Can you work these out from the drawing? Everything is in mm from the part's minimum corner. A direction names the side the tool comes from. Round coordinates to 2 decimals unless told otherwise and drop trailing zeros. Order: outer loops, then holes, each group sorted by start corner. A loop starts at its lowest first (then second) coordinate and runs counter-clockwise, first axis right, second up. Notation, with made-up numbers: (88.5, 17) - (129.5, 17) arc R13 cw to (129.5, 40) - close; hole circle Ø4 at (36.5, 2.25). An arc over 180 degrees is marked (long way). Answer as a JSON object with one key per item and string values.
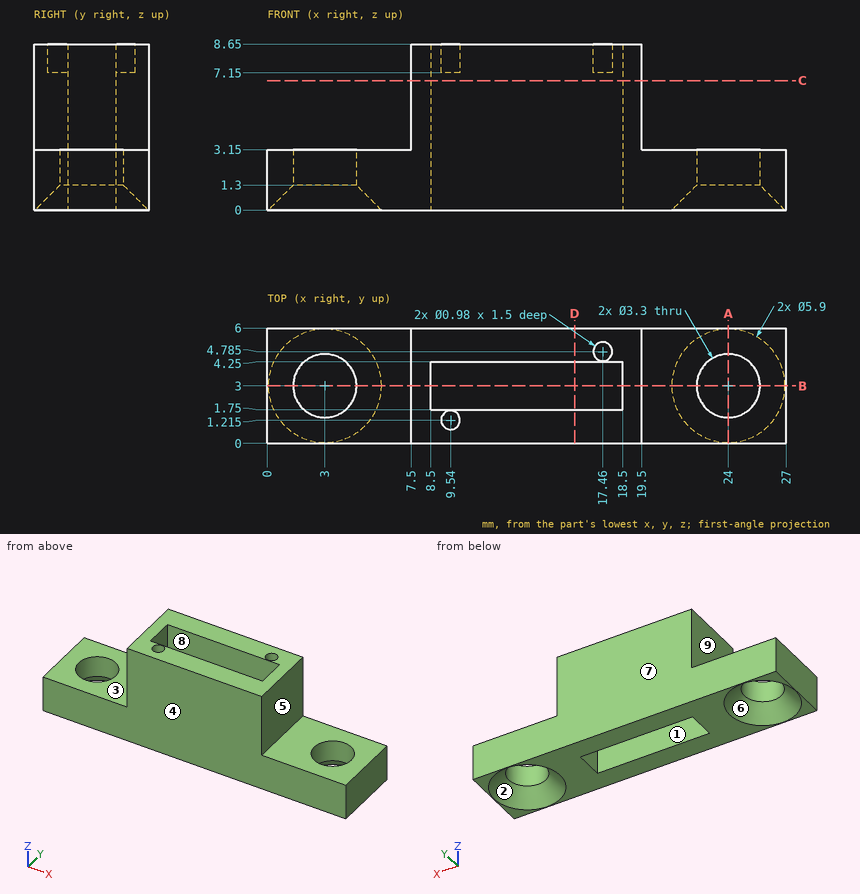
1. For P1, Ø3, axis at x = 22, y = 1.5, coming from the +Z side; P2, Ø1.5, axis at y = 4.5, z = 6, coming from the -X side; P3, Ø2.5, axis at x = 3, y = 3, coming from the -Z side, each with a flat end and sliding along its axis, tell me the tip position at first contact or that it passes through.
Responses:
{"P1": "z = 3.15", "P2": "x = 7.5", "P3": "through"}
2. Imagine slicing it at D-D (x = 16). List the corners of the cut face in (y, z) for me, plus the area to 3 significant figures.
Responses:
{"outline": "(0, 0) - (1.75, 0) - (1.75, 8.65) - (0, 8.65) - close; (4.25, 0) - (6, 0) - (6, 8.65) - (4.25, 8.65) - close", "area": "30.3 mm2"}
3. For the marked faces 1, 2, 3, 4 and 5, which set-ups out of +Z, -Z, +X, -X, +Y, -Y let a thin tool reach every point of the face, with its end or its side?
Responses:
{"face 1": "+Z, -Z", "face 2": "-Z", "face 3": "+Z, -X, +Y, -Y", "face 4": "+Z, -Z, +X, -X, -Y", "face 5": "+Z, +X, +Y, -Y"}
4. Imagine slicing it at A-A (x = 24). List the corners of the cut face in (y, z) for me, plus the area to 4 significant figures.
Responses:
{"outline": "(0, 0) - (0.05, 0) - (1.35, 1.3) - (1.35, 3.15) - (0, 3.15) - close; (4.65, 1.3) - (5.95, 0) - (6, 0) - (6, 3.15) - (4.65, 3.15) - close", "area": "6.815 mm2"}
5. Imagine slicing it at C-C (z = 6.75). List the corners of the cut face in (x, y) for me, plus the area to 3 significant figures.
Responses:
{"outline": "(7.5, 0) - (19.5, 0) - (19.5, 6) - (7.5, 6) - close; hole (8.5, 1.75) - (18.5, 1.75) - (18.5, 4.25) - (8.5, 4.25) - close", "area": "47.0 mm2"}
6. If I drill on L1, parallel to Y at x = 14, z = 2; L2, parallel to Y at x = 24, z = 1.8; L3, parallel to X at y = 2.4, z = 6.5, over which ranges is the centre line in solid material (lowest first)? Write a range as [from, to].
Responses:
{"L1": "[0, 1.75], [4.25, 6]", "L2": "[0, 1.35], [4.65, 6]", "L3": "[7.5, 8.5], [18.5, 19.5]"}
7. Thinking about a two-plate mould opening in Y: for the marked faces 6, 7, 8 and 9, which applies, pulls with the +Y half, pulls with the -Y half, needs draft (parallel to the pull), parting line crosses it, or undercut?
Responses:
{"face 6": "undercut", "face 7": "pulls with the +Y half", "face 8": "undercut", "face 9": "needs draft"}
8. Imagine slicing it at B-B (y = 3). List the corners of the cut face in (x, z) for me.
Responses:
{"outline": "(0, 0) - (0.05, 0) - (1.35, 1.3) - (1.35, 3.15) - (0, 3.15) - close; (4.65, 1.3) - (5.95, 0) - (8.5, 0) - (8.5, 8.65) - (7.5, 8.65) - (7.5, 3.15) - (4.65, 3.15) - close; (18.5, 0) - (21.05, 0) - (22.35, 1.3) - (22.35, 3.15) - (19.5, 3.15) - (19.5, 8.65) - (18.5, 8.65) - close; (25.65, 1.3) - (26.95, 0) - (27, 0) - (27, 3.15) - (25.65, 3.15) - close"}
